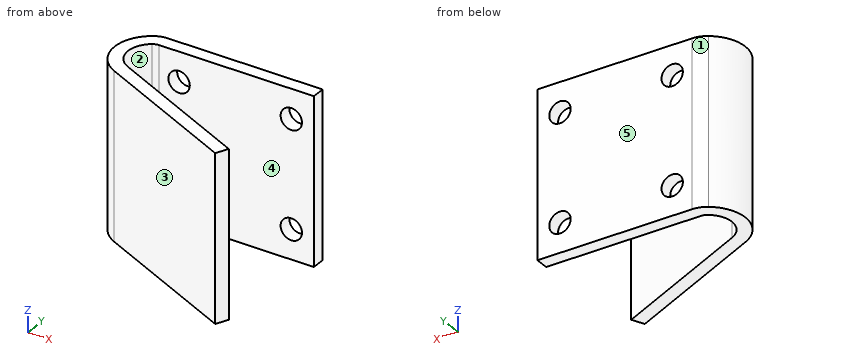
Autodesk Inventor part; units mm, degrees
ref_plane "Work Plane1" through (-1.0565, -14.9443, 31) normal (0, 0, -1) x (0, 1, 0)
ref_plane "YZ Plane" through (0, 0, 0) normal (1, 0, 0) x (0, 1, 0)
ref_plane "XZ Plane" through (0, 0, 0) normal (0, 1, 0) x (-1, 0, 0)
sketch "Sketch1" plane through (0, 0, 0) normal (0, 0, 1) x (1, 0, 0)
  line L0 (0, 0) -> (27.1892, -12.6785)
  line L1 (-1.0565, -2.2658) -> (26.1327, -14.9443)
  line L2 (-1.8478, -3.9627) -> (0.8452, 1.8126)
  line L3 (27.1892, -12.6785) -> (26.1327, -14.9443)
  line L4 (29.393, 8.2928) -> (0.4528, 8.2928)
  arc A0 (-0.6947, 7.9309) -> (0, 0) centre (1.9427, 4.166) ccw
  arc A1 (0.4528, 8.2928) -> (-0.6947, 7.9309) centre (0.4528, 6.2928) ccw
  arc A2 (-2.129, 9.9785) -> (-1.0565, -2.2658) centre (1.9427, 4.166) ccw
  arc A3 (0.4528, 10.7928) -> (-2.129, 9.9785) centre (0.4528, 6.2928) ccw
  line L5 (0.4528, 10.7928) -> (29.393, 10.7928)
  line L6 (29.393, 8.2928) -> (29.393, 10.7928)
  point P0 (-0.082, 8.2928)
  dimension "d2" = 2
ref_plane "Work Plane1" through (-1.0565, -14.9443, 31) normal (0, 0, -1) x (0, 1, 0)
extrude "Extrusion1" add sketch "Sketch1" along normal up to surface (31 mm away)
sketch "Sketch2" plane through (0.4528, 10.7928, 0) normal (0, 1, 0) x (1, 0, 0)
  line L0 (28.9401, 0) -> (28.9401, -31)
  line L1 (0, 0) -> (0, -31)
  line L2 (28.9401, 0) -> (0, 0)
  line L3 (0, 0) -> (0, -15.5)
  line L4 (0, -15.5) -> (28.9401, -15.5)
  line L5 (28.9401, -15.5) -> (28.9401, 0)
  line L6 (24.7213, -15.5) -> (28.7213, -15.5)
  line L7 (24.7213, -15.5) -> (24.7213, -25.5)
  line L8 (24.7213, -25.5) -> (3.7213, -25.5)
  line L9 (3.7213, -25.5) -> (3.7213, -5.5)
  line L10 (3.7213, -5.5) -> (24.7213, -5.5)
  line L11 (24.7213, -5.5) -> (24.7213, -25.5)
  circle A0 centre (24.7213, -5.5) radius 2
  circle A1 centre (24.7213, -25.5) radius 2
  circle A2 centre (3.7213, -25.5) radius 2
  circle A3 centre (3.7213, -5.5) radius 2
  point P0 (-0.4528, 0)
  dimension "d5" = 4
  dimension "d6" = 10
  dimension "d7" = 21
  dimension "d8" = 20
  dimension "d9" = 4
  dimension "d10" = 4
  dimension "d11" = 4
  dimension "d12" = 4
extrude "Extrusion2" cut sketch "Sketch2" against normal up to surface (2.5 mm away) contours A1 L8 L7 | L7 L8 A1 | A0 L10 L11 | L11 L10 A0 | A2 L8 L9 | L9 L8 A2 | A3 L10 L9 | L9 L10 A3
properties part number "helmet_holder"
Work out the finished part from the listing and answer in its coordinate system (mm). Face numbers are marked on the shaded views. A direction names the side the tool comes from. Coordinates: 2 decimals unless noted, no trailing zeros. Write each loop counter-clockwise with the first axis right and the second up, starting at its lowest first coordinate (ties: lowest second). Pieces come first, ordered by that corner, then holes.
1. The part is cut by section C-C, the plane x = 24. Write down the section's boundary in (y, z).
Results list:
outline: (-13.95, 0) - (-11.19, 0) - (-11.19, 31) - (-13.95, 31) - close; (8.29, 0) - (10.79, 0) - (10.79, 3.88) - (8.29, 3.88) - close; (8.29, 7.12) - (10.79, 7.12) - (10.79, 23.88) - (8.29, 23.88) - close; (8.29, 27.12) - (10.79, 27.12) - (10.79, 31) - (8.29, 31) - close
2. The part is cut by section B-B, the plane x = 12. Write down the section's boundary in (y, z).
Results list:
outline: (-8.35, 0) - (-5.6, 0) - (-5.6, 31) - (-8.35, 31) - close; (8.29, 0) - (10.79, 0) - (10.79, 31) - (8.29, 31) - close
3. Flat-ended cylindrical pins translate along their axes: pin 1 (10 mm diameter, centred on x = 10, y = -8.5, fed in from +Z); pin 2 (5 mm diameter, centred on y = 5, z = 11.5, fed in from +X); pin 3 (1 mm diameter, centred on y = -12.5, z = 26.5, fed in from -X); pin 4 (6 mm diameter, centred on x = 7, z = 27.5, fed in from -Y). Find the tip coordinate at first contact, or state that the pin passes through.
Results list:
pin 1: stops at z = 31
pin 2: stops at x = -1.22
pin 3: stops at x = 19.82
pin 4: stops at y = -7.42
4. The part is cut by section D-D, the plane y = 8.75. Write down the section's boundary in (x, z).
Results list:
outline: (-3.47, 0) - (29.39, 0) - (29.39, 31) - (-3.47, 31) - close; hole circle Ø4 at (4.17, 5.5); hole circle Ø4 at (4.17, 25.5); hole circle Ø4 at (25.17, 5.5); hole circle Ø4 at (25.17, 25.5)
5. The part is cut by section A-A, the plane z = 5.5. Write down the section's boundary in (x, y).
Results list:
outline: (-2.13, 9.98) arc R7.1 ccw to (-1.06, -2.27) - (26.13, -14.94) - (27.19, -12.68) - (0, 0) arc R4.6 cw to (-0.69, 7.93) arc R2 cw to (0.45, 8.29) - (2.17, 8.29) - (2.17, 10.79) - (0.45, 10.79) arc R4.5 ccw to start; (6.17, 8.29) - (23.17, 8.29) - (23.17, 10.79) - (6.17, 10.79) - close; (27.17, 8.29) - (29.39, 8.29) - (29.39, 10.79) - (27.17, 10.79) - close
6. For the marked faces 4 and 5, determine the directions among +Z, -Z, +X, -X, +Y, -Y from which every point of the face is accessible in a straight line to the end or side of a thin tool.
Results list:
face 4: +Z, -Z, +X
face 5: +Z, -Z, +X, -X, +Y
7. Consider line 1 along X through (y, z) = (9, 25.5); line 2 along X through (y, z) = (9.7, 5.5); line 3 along Y through (x, z) = (18, 22). Determine where each line is inside the solid, lowest interval first.
Results list:
line 1: x = -3.25 to 2.17, 6.17 to 23.17, 27.17 to 29.39
line 2: x = -2.5 to 2.17, 6.17 to 23.17, 27.17 to 29.39
line 3: y = -11.15 to -8.39, 8.29 to 10.79
8. For a pull along Y with two mould halves and no side action, classify the marked faces 1, 2 and 3 as +Y half, -Y half, draft (parallel to the pull), parting line (faces both ways), or undercut.
Results list:
face 1: +Y half
face 2: undercut
face 3: -Y half
